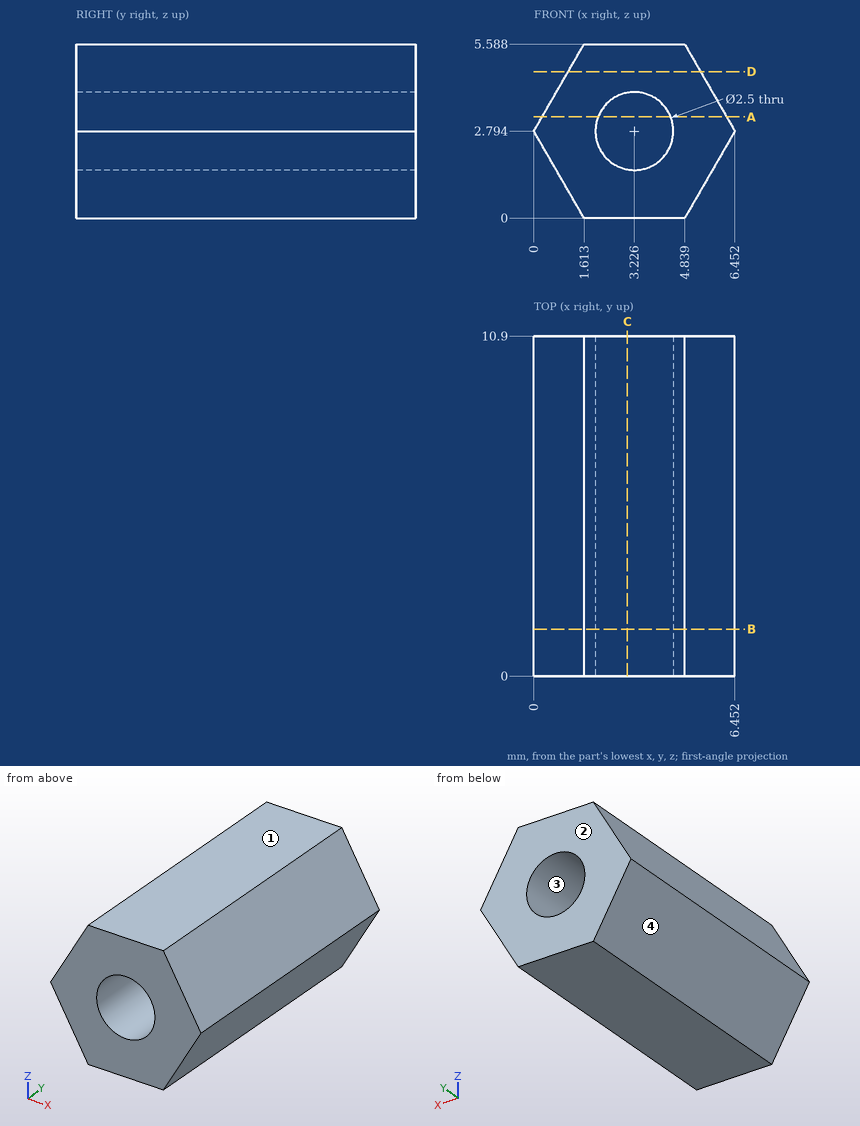
Job drawing, mm, ordinate dimensions from the low corner. One solid piece. Round coordinates to 2 decimals unless told otherwise and drop trailing zeros. Loops run counter-clockwise (first coordinate to the right, second up) from the corner with the lowest first, then second, coordinate; pieces in that order, holes last. Notation, with made-up numbers: (33, -31.5) -> (74, -31.5) arc R18 cw to (74, -16.5) -> close; hole circle Ø11 at (13, 52.25). An arc over 180 degrees is marked (long way). One line per item, written item: value. Start each with the question number.
Q1. Probe line 1 along Z through (x, y) = (3.25, 10.5) (1 decimal); line 2 along X through (y, z) = (4.25, 3.55) (1 decimal); line 3 along X through (y, z) = (4.75, 2.75) (1 decimal). List the from-to ranges inside material, lowest first.
Q2. Two-plate mould, pull along Z, no slides. Class the marked faces 1, 2, 3 and 4: released by +Z, released by -Z, zero draft, split by the parting line, or undercut.
Q3. Cut at A-A on z = 3.25. List the corners of the cut face in (x, y).
Q4. Cut at B-B on y = 1.5. List the corners of the cut face in (x, z).
Q5. Cut at D-D on z = 4.7. List the corners of the cut face in (x, y).
Q6. Cut at C-C on x = 3. List the corners of the cut face in (y, z) (1 decimal).
Computed:
1. line 1: 0 to 1.5, 4 to 5.6
1. line 2: 0.4 to 2.2, 4.2 to 6
1. line 3: 0 to 2, 4.5 to 6.4
2. face 1: released by +Z
2. face 2: zero draft
2. face 3: undercut
2. face 4: released by -Z
3. outline: (0.26, 0) -> (2.06, 0) -> (2.06, 10.9) -> (0.26, 10.9) -> close; (4.39, 0) -> (6.19, 0) -> (6.19, 10.9) -> (4.39, 10.9) -> close
4. outline: (0, 2.79) -> (1.61, 0) -> (4.84, 0) -> (6.45, 2.79) -> (4.84, 5.59) -> (1.61, 5.59) -> close; hole circle Ø2.5 at (3.23, 2.79)
5. outline: (1.1, 0) -> (5.35, 0) -> (5.35, 10.9) -> (1.1, 10.9) -> close
6. outline: (0, 0) -> (10.9, 0) -> (10.9, 1.6) -> (0, 1.6) -> close; (0, 4) -> (10.9, 4) -> (10.9, 5.6) -> (0, 5.6) -> close
